from build123d import *

# Parameters (mm, degrees)
CUT_EXTRUDE1_DEPTH  = 56.621758333
CIRPATTERN1_COUNT   = 4
SKETCH3_R           = 23.75
CUT_EXTRUDE2_DEPTH  = 12
CUT_EXTRUDE3_START  = 12
CUT_EXTRUDE3_DEPTH  = 12
CIRPATTERN2_COUNT   = 4
SKETCH5_R           = 5
SKETCH5_R_2         = 2.35
BOSS_EXTRUDE1_DEPTH = 14
CHAMFER1_SIZE       = 1
CHAMFER2_SIZE       = 5


with BuildPart() as part:
    # Sketch1 → Revolve1 (revolve)
    with BuildSketch(Plane(origin=(0, 0, 0), x_dir=(0, 0, -1), z_dir=(1, 0, 0)), mode=Mode.PRIVATE) as revolve1_sk:
        Polygon((0, 0), (26.7, 0), (26.7, 18), (36.7, 18), (36.7, 20), (0, 20), align=None)
    revolve(revolve1_sk.sketch.rotate(Axis((0, 20, 0), (0, -1, 0)), 180), axis=Axis((0, 20, 0), (0, -1, 0)))

    # Sketch2 → Cut-Extrude1 (cut, symmetric)
    with BuildSketch(Plane.XY):
        Polygon((4.121320344, 20), (0, 15.878679656), (-4.121320344, 20), align=None)
    cut_extrude1 = extrude(amount=CUT_EXTRUDE1_DEPTH, both=True, mode=Mode.SUBTRACT)

    # CirPattern1: Cut-Extrude1 ×4 about axis
    cirpattern1_axis = Axis((0, 0, 0), (0, 1, 0))
    for i in range(1, CIRPATTERN1_COUNT):
        add(cut_extrude1.rotate(cirpattern1_axis, i * 360 / CIRPATTERN1_COUNT), mode=Mode.SUBTRACT)

    # Sketch3 → Cut-Extrude2 (cut)
    with BuildSketch(Plane.XZ):
        with Locations(Location((0, 0, 0), (0, 0, 270))):
            Circle(SKETCH3_R)
    extrude(amount=-CUT_EXTRUDE2_DEPTH, mode=Mode.SUBTRACT)

    # Sketch4 → Cut-Extrude3 (cut)
    with BuildSketch(Plane(origin=(0, 0, 0), x_dir=(1, 0, 0), z_dir=(0, 1, 0)).offset(CUT_EXTRUDE3_START)):
        with BuildLine():
            Line((-25.234076692, -26.648290255), (0, -1.414213562))
            Line((0, -1.414213562), (-1.414213562, 0))
            Line((-1.414213562, 0), (-26.648290255, -25.234076692))
            ThreePointArc((-26.648290255, -25.234076692), (-25.95081887, -25.95081887), (-25.234076692, -26.648290255))
        make_face()
    cut_extrude3 = extrude(amount=-CUT_EXTRUDE3_DEPTH, mode=Mode.SUBTRACT)

    # CirPattern2: Cut-Extrude3 ×4 about axis
    cirpattern2_axis = Axis((0, 0, 0), (0, 1, 0))
    for i in range(1, CIRPATTERN2_COUNT):
        add(cut_extrude3.rotate(cirpattern2_axis, i * 360 / CIRPATTERN2_COUNT), mode=Mode.SUBTRACT)

    # Sketch5 → Boss-Extrude1 (add)
    with BuildSketch(Plane.XZ.offset(-12)):
        with Locations(Location((0, 0, 0), (0, 0, 270))):
            Circle(SKETCH5_R)
        with Locations(Location((0, 0, 0), (0, 0, 270))):
            Circle(SKETCH5_R_2, mode=Mode.SUBTRACT)
    extrude(amount=BOSS_EXTRUDE1_DEPTH)

    # Chamfer1
    chamfer1_edges = [part.edges().sort_by_distance(p)[0] for p in [
        (0, -2, 2.35),
    ]]
    chamfer(chamfer1_edges, length=CHAMFER1_SIZE)

    # Chamfer2
    chamfer2_edges = [part.edges().sort_by_distance(p)[0] for p in [
        (0, 12, 5),
    ]]
    chamfer(chamfer2_edges, length=CHAMFER2_SIZE)


solid = part.part
Geometry: final body of the model. Coordinates: model frame, mm. A direction names the side the tool comes from. Round coordinates to 2 decimals unless told otherwise and drop trailing zeros. Write each loop counter-clockwise with the first axis right and the second up, starting at its lowest first coordinate (ties: lowest second). Pieces come first, ordered by that corner, then holes. Notation, with made-up numbers: M 4.5,39 L 29.5,39 A21 ccw 29.5,56 Z; hole C 73,7 d1. An arc over 180 degrees is marked long. Write item = value, one per line.
Item 1: Pin query (flat end, axial travel): P1, Ø5, axis at x = -1, z = 1, coming from the -Y side; P2, Ø6, axis at x = -23, z = 4, coming from the -Y side; P3, Ø6, axis at x = 0, z = 0, coming from the -Y side; P4, Ø1, axis at y = 12, z = -18.5, coming from the -X side. Return the tip coordinate at first contact, or that it passes through.
Findings:
P1 = -2
P2 = 0
P3 = -1.65
P4 = -19.72
Item 2: Section query A-A on y = 3.75. Return loops of the section in (x, z), then the cut area to 3 significant figures.
Findings:
outline = M -19.57,-18.16 L -17.49,-16.07 A23.75 cw -17.49,16.07 L -19.57,18.16 A26.7 ccw Z; M -18.16,-19.57 A26.7 ccw 18.16,-19.57 L 16.07,-17.49 A23.75 cw -16.07,-17.49 Z; M -18.16,19.57 L -16.07,17.49 A23.75 cw 16.07,17.49 L 18.16,19.57 A26.7 ccw Z; C 0,0 d10; M 17.49,-16.07 L 19.57,-18.16 A26.7 ccw 19.57,18.16 L 17.49,16.07 A23.75 cw Z; hole C 0,0 d4.7
area = 505 mm^2
Item 3: Section query C-C on x = 13. Return loops of the section in (y, z), then the cut area to 3 significant figures.
Findings:
outline = M 0,-23.32 L 18,-23.32 L 18,-34.32 L 20,-34.32 L 20,-4.12 L 15.88,0 L 20,4.12 L 20,34.32 L 18,34.32 L 18,23.32 L 0,23.32 L 0,19.88 L 12,19.88 L 12,-19.88 L 0,-19.88 Z
area = 483 mm^2
Item 4: Access query for faces 1 (the face through (18.58, 17.91, 2.03)), 2 (the face through (18.515, 6.084, -17.101)), 3 (the face through (-2.03, 17.91, -18.06)), 4 (the face through (1, 0, -24)). Directions: +Z, -Z, +X, -X, +Y, -Y. A direction counts if a zero-diameter tool reaches every point of the face in a straight line with its end or side. Return the directions, or none.
Findings:
face_1 = +X, -X, +Y
face_2 = -Y
face_3 = +Z, -Z, +Y
face_4 = -Z, +X, -X, -Y
Item 5: Section query D-D on z = -31.5. Return loops of the section in (x, y).
Findings:
outline = M -18.83,18 L -2.12,18 L -4.12,20 L -18.83,20 Z; M 2.12,18 L 18.83,18 L 18.83,20 L 4.12,20 Z
Item 6: Material intervals for line 1 along X through (y, z) = (5.5, 0); line 2 along X through (y, z) = (7.75, 0); line 3 along Y through (x, z) = (17.5, -22), sorted ascending. Write a range as [from, to].
Findings:
line_1 = [-26.7, -23.75], [-5, -2.35], [2.35, 5], [23.75, 26.7]
line_2 = [-26.7, -23.75], [-5.75, -2.35], [2.35, 5.75], [23.75, 26.7]
line_3 = [18, 20]
Item 7: Section query B-B on z = 29. Return loops of the section in (x, y), then the cut area to 3 significant figures.
Findings:
outline = M -22.49,18 L -2.12,18 L -4.12,20 L -22.49,20 Z; M 2.12,18 L 22.49,18 L 22.49,20 L 4.12,20 Z
area = 77.5 mm^2
